```python
from build123d import *

# Parameters (mm, degrees)
SKETCH1_W           = 3.175
SKETCH1_H           = 28.575
BOSS_EXTRUDE1_DEPTH = 76.2
SKETCH2_R           = 3.175
CUT_EXTRUDE1_DEPTH  = 76.2


with BuildPart() as part:
    # Sketch1 → Boss-Extrude1 (new body)
    with BuildSketch(Plane(origin=(0, 0, 0), x_dir=(0, 0, -1), z_dir=(1, 0, 0))):
        with Locations((-1.5875, 14.2875)):
            Rectangle(SKETCH1_W, SKETCH1_H)
        Polygon((28.575, 0), (0, 0), (-3.175, 0), (-3.175, -3.175), (28.575, -3.175), align=None)
    extrude(amount=BOSS_EXTRUDE1_DEPTH)

    # Sketch2 → Cut-Extrude1 (cut)
    with BuildSketch(Plane(origin=(0, 0, 0), x_dir=(-1, 0, 0), z_dir=(0, 0, -1))):
        with Locations((-38.1, 15.875)):
            Circle(SKETCH2_R)
        with Locations((-63.5, 15.875)):
            Circle(SKETCH2_R)
        with Locations((-12.7, 15.875)):
            Circle(SKETCH2_R)
    extrude(amount=-CUT_EXTRUDE1_DEPTH, mode=Mode.SUBTRACT)


solid = part.part
```
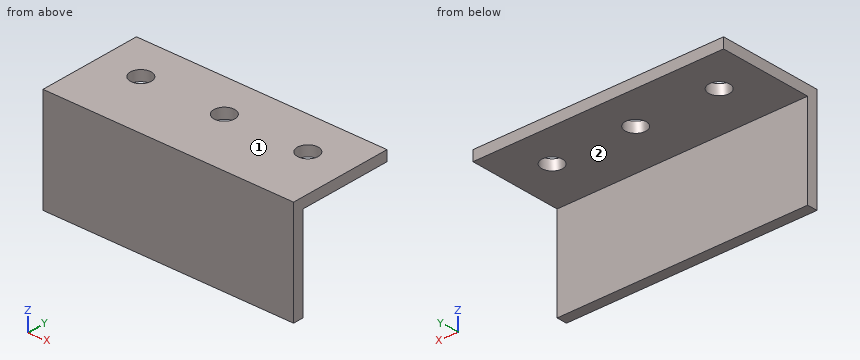
Verification items for the finished model (mm, model axes). Face numbers are marked on the shaded views. A direction names the side the tool comes from. Give positions to 0.01 mm unless a question says otherwise; leave off trailing zeros. Order: outer loops, then holes, each group sorted by start corner. A loop starts at its lowest first (then second) coordinate and runs counter-clockwise, first axis right, second up. Notation, with made-up numbers: M 29.5,-31 L 40.5,-31 A21 ccw 40.5,-22 Z; hole C 44,29 d4. An arc over 180 degrees is marked long. Return JSON: item names as keys, results as strings. Group by question number.
1) Access from +Z, -Z, +X, -X, +Y, -Y to the whole of each face (thin tool, end or side, straight path). Record for the marked faces 1 and 2.
2) Section check D-D on z = -22. Record the cut outline in (x, y) (3 decimals).
3) Scan lines: line 1 (Y direction, x = 38, z = 2) (3 decimals); line 2 (Z direction, x = 8.5, y = 7.5) (3 decimals); line 3 (Y direction, x = 28, z = -23) (3 decimals). Record each from-to range of solid material in increasing order.
4) Section check B-B on x = 55. Record the cut outline in (y, z) (3 decimals).
5) Section check C-C on y = 26.5. Record the cut outline in (x, z) (3 decimals), and give its area (3 significant figures).
6) Go/stop test with flat-tipped pins: pin 1 Ø8.5 at (x, y) = (38.1, 15.875) entering from -Z; pin 2 Ø2 at (x, z) = (18, -16.5) entering from +Y. Record where each tip stops, or that it passes through.
7) Section check A-A on x = 12.7. Record the cut outline in (y, z) (3 decimals).
Answer block:
{
 "1": {"face 1": "+Z, +X, -X, +Y, -Y", "face 2": "-Z, +X, -X, +Y"},
 "2": {"outline": "M 0,-3.175 L 76.2,-3.175 L 76.2,0 L 0,0 Z"},
 "3": {"line 1": "y = -3.175 to 12.702, 19.048 to 28.575", "line 2": "z = 0 to 3.175", "line 3": "y = -3.175 to 0"},
 "4": {"outline": "M -3.175,-28.575 L 0,-28.575 L 0,0 L 28.575,0 L 28.575,3.175 L -3.175,3.175 Z"},
 "5": {"outline": "M 0,0 L 76.2,0 L 76.2,3.175 L 0,3.175 Z", "area": "242 mm^2"},
 "6": {"pin 1": "stops at z = 0", "pin 2": "stops at y = 0"},
 "7": {"outline": "M -3.175,-28.575 L 0,-28.575 L 0,0 L 12.7,0 L 12.7,3.175 L -3.175,3.175 Z; M 19.05,0 L 28.575,0 L 28.575,3.175 L 19.05,3.175 Z"}
}
